from build123d import *

# Parameters (mm, degrees)
SKETCH001_W                          = 2
SKETCH001_H                          = 6
EXTRUDE002_DEPTH                     = 1
SKETCH002_AS_DRAWN_R                 = 3.025
EXTRUDE001_DEPTH                     = 100
EXTRUDE001_ONTO_SKETCH002_ROLL_ANGLE = 90
EXTRUDE_DEPTH                        = 17
FILLET_R                             = 1
FILLET001_R                          = 3
FILLET002_R                          = 1.5


with BuildPart() as extrude002:
    # Sketch001 → Extrude002 (new body)
    with BuildSketch(Plane.XY.offset(17)):
        with Locations((16.997575, 23.384003)):
            Rectangle(SKETCH001_W, SKETCH001_H)
        with Locations((21.997575, 23.384003)):
            Rectangle(SKETCH001_W, SKETCH001_H)
        with Locations((26.997575, 23.384003)):
            Rectangle(SKETCH001_W, SKETCH001_H)
    extrude(amount=EXTRUDE002_DEPTH)


with BuildPart() as extrude001:
    # Sketch002 as drawn → Extrude001 (new)
    with BuildSketch(Plane.XY):
        with Locations((22, 8.5)):
            Circle(SKETCH002_AS_DRAWN_R)
    extrude(amount=-EXTRUDE001_DEPTH)


with BuildPart() as extrude001_1:
    # Extrude001 onto Sketch002 roll: moved
    add(extrude001.part.rotate(Axis((0, 0, 0), (1, 0, 0)), EXTRUDE001_ONTO_SKETCH002_ROLL_ANGLE))


with BuildPart() as extrude001_2:
    # Extrude001 onto Sketch002 placement: moved
    add(extrude001_1.part)


with BuildPart() as fusion:
    # Sketch → Extrude (new body)
    with BuildSketch(Plane.XY):
        with BuildLine():
            Line((4.638368, 11.639512), (9.638368, 11.639512))
            ThreePointArc((34.356782, 11.639512), (21.997575, 18.139512), (9.638368, 11.639512))
            Line((34.356782, 11.639512), (39.356782, 11.639512))
            Line((39.356782, 11.639512), (39.356782, 14.139512))
            Line((39.356782, 14.139512), (35.821248, 17.675046))
            Line((35.821248, 17.675046), (40.736161, 21.116505))
            Line((40.736161, 21.116505), (47.709524, 21.726595))
            ThreePointArc((47.709524, 21.726595), (43.383687, 27.276008), (37.792049, 23.004892))
            Line((37.792049, 23.004892), (35.822433, 23.352189))
            ThreePointArc((35.822433, 23.352189), (20.558831, 30.621918), (8.221554, 19.062589))
            ThreePointArc((8.221554, 19.062589), (6.928179, 17.283763), (6.638368, 15.103614))
            Line((4.638368, 11.639512), (6.638368, 15.103614))
        make_face()
    extrude(amount=EXTRUDE_DEPTH)

    # Fillet
    fillet_edges = [fusion.edges().sort_by_distance(p)[0] for p in [
        (4.638368, 11.639512, 8.5),
        (9.638368, 11.639512, 8.5),
        (47.709524, 21.726595, 8.5),
        (37.792049, 23.004892, 8.5),
        (35.822433, 23.352189, 8.5),
    ]]
    fillet(fillet_edges, radius=FILLET_R)

    # Fillet001
    fillet001_edges = [fusion.edges().sort_by_distance(p)[0] for p in [
        (34.356782, 11.639512, 8.5),
        (39.356782, 14.139512, 8.5),
    ]]
    fillet(fillet001_edges, radius=FILLET001_R)

    # Fillet002
    fillet002_edges = [fusion.edges().sort_by_distance(p)[0] for p in [
        (39.356782, 11.639512, 8.5),
    ]]
    fillet(fillet002_edges, radius=FILLET002_R)

    # Cut: cut Extrude001
    add(extrude001_2.part, mode=Mode.SUBTRACT)

    # Fusion: union Extrude002
    add(extrude002.part)


solid = fusion.part
Geometry: final body of the model. Coordinates: model frame, mm. A direction names the side the tool comes from. Coordinates: 2 decimals unless noted, no trailing zeros. Order: outer loops, then holes, each group sorted by start corner. A loop starts at its lowest first (then second) coordinate and runs counter-clockwise, first axis right, second up.
(1) Access query for faces 5 (the face through (9.568, 11.744, 8.619)), 6 (the face through (17, 20.384, 17.5)), 7 (the face through (17, 26.384, 17.5)), 8 (the face through (20.998, 23.3, 17.5)). Directions: +Z, -Z, +X, -X, +Y, -Y. A direction counts if a zero-diameter tool reaches every point of the face in a straight line with its end or side. Return the directions, or none.
(2) Draft query along Y for faces 1 (the face through (38.24, 19.37, 8.38)), 2 (the face through (27.998, 23.3, 17.5)), 3 (the face through (37.168, 16.328, 8.381)), 4 (the face through (5.51, 12.13, 8.62)). Return one class per face: pulls with the +Y half, pulls with the -Y half, needs draft (parallel to the pull), parting line crosses it, or undercut.
(3) Section query B-B (y = 28). Return the cut outline in (x, z) (3 decimals), plus the area to 3 significant figures.
(4) Section query A-A (x = 22). Return the cut outline in (y, z) (3 decimals), plus the area to 3 significant figures.
(5) Material intervals for probe 1 along Z at (x, y) = (22, 24) (3 decimals); probe 2 along X at (y, z) = (24, 8.5) (3 decimals); probe 3 along Z at (x, y) = (22, 26.75) (3 decimals), sorted ascending.
(6) First-contact query: pin 1 (8 mm diameter, centred on x = 30, z = 8, fed in from -Y); pin 2 (0.8 mm diameter, centred on x = 17.5, z = 17.5, fed in from -Y); pin 3 (0.5 mm diameter, centred on y = 23.5, z = 17.5, fed in from -X). Flat tips, straight axial feed; report the tip coordinate or a pass-through.
(7) Section query D-D (y = 19.5). Return the cut outline in (x, z) (3 decimals), plus the area to 3 significant figures.
(8) Section query C-C (x = 11). Return the cut outline in (y, z), plus the area to 3 significant figures.
Solution:
1. face 5: +Z, -Z, -Y
1. face 6: +Z, +X, -X, -Y
1. face 7: +Z, +X, -X, +Y
1. face 8: +Z, +Y, -Y
2. face 1: undercut
2. face 2: needs draft
2. face 3: undercut
2. face 4: parting line crosses it
3. outline: (14.136, 0) - (31.589, 0) - (31.589, 17) - (14.136, 17) - close; hole circle Ø6.05 at (22, 8.5)
3. area: 268 mm2
4. outline: (18.14, 0) - (30.775, 0) - (30.775, 5.475) - (18.14, 5.475) - close; (18.14, 11.525) - (30.775, 11.525) - (30.775, 17) - (26.384, 17) - (26.384, 18) - (20.384, 18) - (20.384, 17) - (18.14, 17) - close
4. area: 144 mm2
5. probe 1: z = 0 to 5.475, 11.525 to 18
5. probe 2: x = 10.302 to 18.975, 25.025 to 35.423, 38.036 to 47.453
5. probe 3: z = 0 to 5.475, 11.525 to 17
6. pin 1: stops at y = 12.27
6. pin 2: stops at y = 20.38
6. pin 3: stops at x = 16
7. outline: (8.326, 0) - (38.428, 0) - (38.428, 17) - (8.326, 17) - close; hole circle Ø6.05 at (22, 8.5)
7. area: 483 mm2
8. outline: (13.34, 0) - (24.98, 0) - (24.98, 17) - (13.34, 17) - close
8. area: 198 mm2
